from build123d import *

# Parameters (mm, degrees)
SKETCH1_R           = 10
SKETCH1_R_2         = 1.397
BOSS_EXTRUDE2_DEPTH = 5.1


with BuildPart() as part:
    # Sketch1 → Boss-Extrude2 (new body)
    with BuildSketch(Plane(origin=(0, 0, 0), x_dir=(1, 0, 0), z_dir=(0, 1, 0))):
        with Locations(Location((0, 0, 0), (0, 0, 270))):
            Circle(SKETCH1_R)
        with BuildLine():
            Line((-1.5, 2), (1.5, 2))
            ThreePointArc((1.5, 2), (0, -2.5), (-1.5, 2))
        make_face(mode=Mode.SUBTRACT)
        with Locations(Location((-6.35, 0, 0), (0, 0, 270))):
            Circle(SKETCH1_R_2, mode=Mode.SUBTRACT)
        with Locations(Location((0, -6.35, 0), (0, 0, 270))):
            Circle(SKETCH1_R_2, mode=Mode.SUBTRACT)
        with Locations(Location((0, 6.35, 0), (0, 0, 270))):
            Circle(SKETCH1_R_2, mode=Mode.SUBTRACT)
        with Locations(Location((6.35, 0, 0), (0, 0, 270))):
            Circle(SKETCH1_R_2, mode=Mode.SUBTRACT)
    extrude(amount=BOSS_EXTRUDE2_DEPTH)


solid = part.part
Can you work these out from the model? Positions are in its coordinate system, mm. A direction names the side the tool comes from. Give positions to 0.01 mm unless a question says otherwise; leave off trailing zeros. Loops run counter-clockwise (first coordinate to the right, second up) from the corner with the lowest first, then second, coordinate; pieces in that order, holes last. Notation, with made-up numbers: (-32, 29.25) -> (20, 29.25) arc R35 ccw to (20, 66.25) -> close; hole circle Ø4 at (29, 66.25). An arc over 180 degrees is marked (long way). Return JSON: item names as keys, results as strings.
Q1. We'd pull the mould along Z, two halves only. Please class faces 1 (the face through (-4.965, 2.514, -0.182)), 2 (the face through (-9.76, 2.51, -2.17)), 3 (the face through (0.1, 0, -2.4)): released by +Z, released by -Z, zero draft, split by the parting line, or undercut.
Checks:
{"face 1": "undercut", "face 2": "split by the parting line", "face 3": "zero draft"}
Q2. On a 3-axis mill with a long thin cutter (end or side, diameter ignored), from which of +Z, -Z, +X, -X, +Y, -Y can I reach the whole of each face in a straight line? I mean faces 4 (the face through (0.1, 5.1, -2.4)), 5 (the face through (0, 3, -2)). Say none if no direction works.
Checks:
{"face 4": "+Z, -Z, +X, -X, +Y", "face 5": "+Y, -Y"}
Q3. I want a section at B-B, the plane z = -6.35. List the corners of the cut face in (x, y) for me, then the cut area to 3 significant figures.
Checks:
{"outline": "(-7.73, 0) -> (-1.4, 0) -> (-1.4, 5.1) -> (-7.73, 5.1) -> close; (1.4, 0) -> (7.73, 0) -> (7.73, 5.1) -> (1.4, 5.1) -> close", "area": "64.5 mm2"}
Q4. For pin 1 Ø2.5 at (x, z) = (-6.35, 0) entering from -Y; pin 2 Ø2 at (x, y) = (7.5, 3.5) entering from +Z, each with a flat end and sliding along its axis, tell me the tip position at first contact or that it passes through.
Checks:
{"pin 1": "passes through", "pin 2": "stops at z = 7.6"}
Q5. I want a section at D-D, the plane x = -6.35. List the corners of the cut face in (y, z) for me, then the cut area to 3 significant figures.
Checks:
{"outline": "(0, -7.73) -> (5.1, -7.73) -> (5.1, -1.4) -> (0, -1.4) -> close; (0, 1.4) -> (5.1, 1.4) -> (5.1, 7.73) -> (0, 7.73) -> close", "area": "64.5 mm2"}
Q6. I need wall thicknesses on probe 1 along X at (y, z) = (2.2, 0); probe 2 along X at (y, z) = (4.3, -1); probe 3 along Z at (x, y) = (1, 3.1). Which ranges of each line are inside material? Lowest first, please.
Checks:
{"probe 1": "x = -10 to -7.75, -4.95 to -2.5, 2.5 to 4.95, 7.75 to 10", "probe 2": "x = -9.95 to -7.33, -5.37 to -2.29, 2.29 to 5.37, 7.33 to 9.95", "probe 3": "z = -9.95 to -7.33, -5.37 to -2, 2.29 to 5.37, 7.33 to 9.95"}
Q7. I want a section at A-A, the plane x = 0. List the corners of the cut face in (y, z) for me, then the cut area to 3 significant figures.
Checks:
{"outline": "(0, -10) -> (5.1, -10) -> (5.1, -7.75) -> (0, -7.75) -> close; (0, -4.95) -> (5.1, -4.95) -> (5.1, -2) -> (0, -2) -> close; (0, 2.5) -> (5.1, 2.5) -> (5.1, 4.95) -> (0, 4.95) -> close; (0, 7.75) -> (5.1, 7.75) -> (5.1, 10) -> (0, 10) -> close", "area": "50.6 mm2"}
Q8. I want a section at C-C, the plane y = 3.25. List the corners of the cut face in (x, z) for me, then the cut area to 3 significant figures.
Checks:
{"outline": "circle Ø20 at (0, 0); hole circle Ø2.79 at (-6.35, 0); hole (-1.5, -2) -> (1.5, -2) arc R2.5 ccw (long way) to start; hole circle Ø2.79 at (0, -6.35); hole circle Ø2.79 at (0, 6.35); hole circle Ø2.79 at (6.35, 0)", "area": "271 mm2"}
